Verification items for this drawing (mm, ordinates from the low corner). Round coordinates to 2 decimals unless told otherwise and drop trailing zeros. Loops run counter-clockwise (first coordinate to the right, second up) from the corner with the lowest first, then second, coordinate; pieces in that order, holes last. Notation, with made-up numbers: (13, 88) - (33, 88) arc R15 ccw to (33, 97) - close; hole circle Ø6 at (14, -15.75). An arc over 180 degrees is marked (long way). Use a Markdown table: item, result. Add a question column.
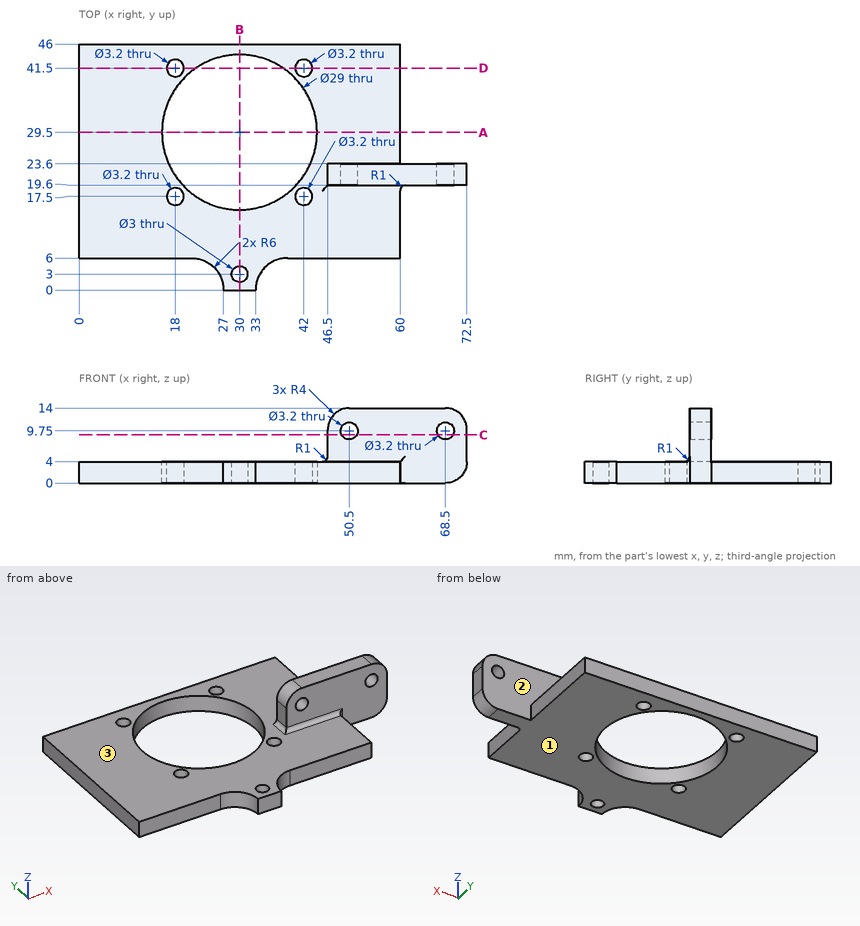
Q1. Section check A-A on y = 29.5. Record the cut outline in (x, z).
Q2. Release check for a two-part mould opening along Z. For the marked faces 1, 2 and 3 record: +Z half, -Z half, draft (parallel to the pull), parting line (faces both ways), or undercut.
Q3. Section check D-D on y = 41.5. Record the cut outline in (x, z).
Q4. Go/stop test with flat-tipped pins: pin 1 Ø2 at (y, z) = (22.5, 8) entering from -X; pin 2 Ø3 at (y, z) = (29.5, 4.5) entering from -X; pin 3 Ø5 at (x, y) = (18, 41.5) entering from +Z; pin 4 Ø1.9 at (x, z) = (50.5, 9.75) entering from +Y. Record where each tip stops, or that it passes through.
Q5. Section check B-B on x = 30. Record the cut outline in (y, z).
Q6. Thickness scan on line 1 along Y through (x, z) = (30, 2.7); line 2 along X through (y, z) = (21.45, 9.75); line 3 along Z through (x, y) = (53.5, 31.5). Record the ranges inside material, lowest first.
Q7. Section check C-C on z = 9. Record the cut outline in (x, y), plus the area to 3 significant figures.
Determined:
| question | item | result |
|---|---|---|
| 1 | outline | (0, 0) - (15.5, 0) - (15.5, 4) - (0, 4) - close; (44.5, 0) - (60, 0) - (60, 4) - (44.5, 4) - close |
| 2 | face 1 | -Z half |
| 2 | face 2 | draft |
| 2 | face 3 | +Z half |
| 3 | outline | (0, 0) - (16.4, 0) - (16.4, 4) - (0, 4) - close; (19.6, 0) - (21.86, 0) - (21.86, 4) - (19.6, 4) - close; (38.14, 0) - (40.4, 0) - (40.4, 4) - (38.14, 4) - close; (43.6, 0) - (60, 0) - (60, 4) - (43.6, 4) - close |
| 4 | pin 1 | stops at x = 46.5 |
| 4 | pin 2 | stops at x = 0 |
| 4 | pin 3 | stops at z = 4 |
| 4 | pin 4 | passes through |
| 5 | outline | (0, 0) - (1.5, 0) - (1.5, 4) - (0, 4) - close; (4.5, 0) - (15, 0) - (15, 4) - (4.5, 4) - close; (44, 0) - (46, 0) - (46, 4) - (44, 4) - close |
| 6 | line 1 | y = 0 to 1.5, 4.5 to 15, 44 to 46 |
| 6 | line 2 | x = 46.5 to 48.9, 52.1 to 66.9, 70.1 to 72.5 |
| 6 | line 3 | z = 0 to 4 |
| 7 | outline | (46.5, 19.6) - (49.09, 19.6) - (49.09, 23.6) - (46.5, 23.6) - close; (51.91, 19.6) - (67.09, 19.6) - (67.09, 23.6) - (51.91, 23.6) - close; (69.91, 19.6) - (72.5, 19.6) - (72.5, 23.6) - (69.91, 23.6) - close |
| 7 | area | 81.4 mm² |
